Verification items for this drawing (mm, ordinates from the low corner). Give positions to 0.01 mm unless a question says otherwise; leave off trailing zeros. Loops run counter-clockwise (first coordinate to the right, second up) from the corner with the lowest first, then second, coordinate; pieces in that order, holes last. Notation, with made-up numbers: (32, 51) -> (45, 51) arc R30 cw to (45, 79) -> close; hole circle Ø7 at (45, 82). An arc over 180 degrees is marked (long way). Write item = value, one per line.
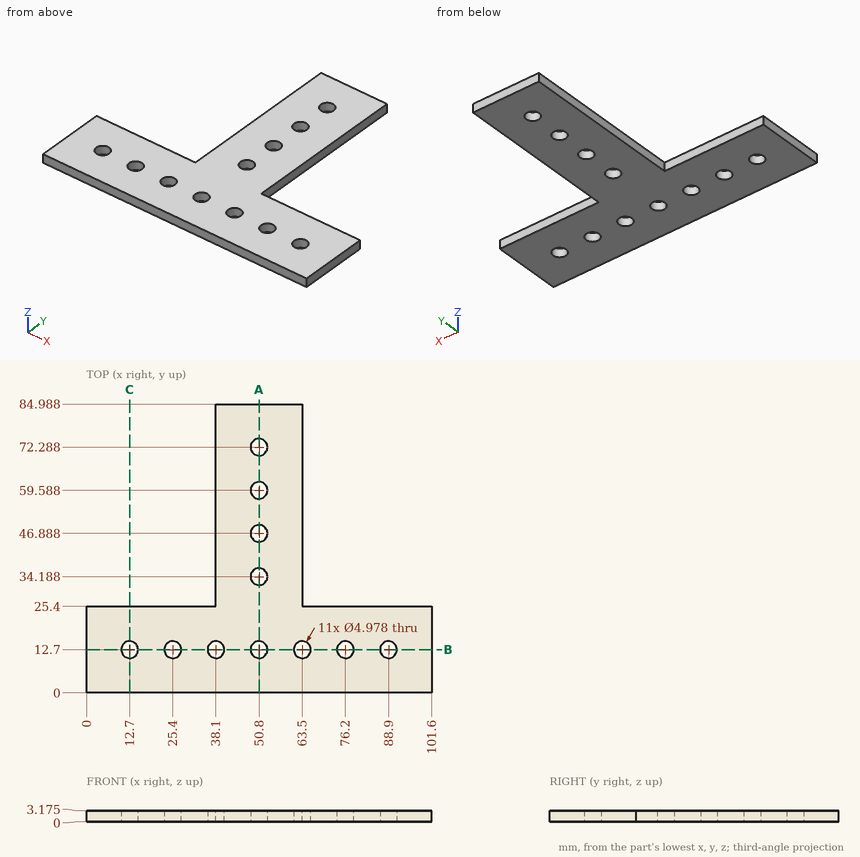
Item 1: Gauge pin test, flat ends, axial feed: pin 1 (1.6 mm diameter, centred on x = 84.5, z = 1.5, fed in from +Y); pin 2 (1 mm diameter, centred on y = 40.5, z = 2, fed in from +X); pin 3 (1 mm diameter, centred on y = 53, z = 1, fed in from -X). Record the tip position at first contact, or that the pin passes through.
Answer:
pin_1 = 25.4
pin_2 = 63.5
pin_3 = 38.1
Item 2: Section check B-B, the plane y = 12.7. Give the number of separate pieces and of enclosed holes in the cut face, plus the area to 3 significant figures.
Answer:
separate_pieces = 8
enclosed_holes = 0
area = 212 mm^2
Item 3: Section check C-C, the plane x = 12.7. Record the cut outline in (y, z) (1 decimal).
Answer:
outline = (0, 0) -> (10.2, 0) -> (10.2, 3.2) -> (0, 3.2) -> close; (15.2, 0) -> (25.4, 0) -> (25.4, 3.2) -> (15.2, 3.2) -> close
Item 4: Section check A-A, the plane x = 50.8. Record the cut outline in (y, z) (1 decimal), plus the area to 3 significant figures.
Answer:
outline = (0, 0) -> (10.2, 0) -> (10.2, 3.2) -> (0, 3.2) -> close; (15.2, 0) -> (31.7, 0) -> (31.7, 3.2) -> (15.2, 3.2) -> close; (36.7, 0) -> (44.4, 0) -> (44.4, 3.2) -> (36.7, 3.2) -> close; (49.4, 0) -> (57.1, 0) -> (57.1, 3.2) -> (49.4, 3.2) -> close; (62.1, 0) -> (69.8, 0) -> (69.8, 3.2) -> (62.1, 3.2) -> close; (74.8, 0) -> (85, 0) -> (85, 3.2) -> (74.8, 3.2) -> close
area = 191 mm^2
Item 5: Thickness scan on L1, parallel to Y at x = 12.7, z = 2.25; L2, parallel to X at y = 80, z = 1.1; L3, parallel to Y at x = 87, z = 3. Record the ranges inside material, lowest first. Write a range as [from, to].
Answer:
L1 = [0, 10.21], [15.19, 25.4]
L2 = [38.1, 63.5]
L3 = [0, 11.09], [14.31, 25.4]
